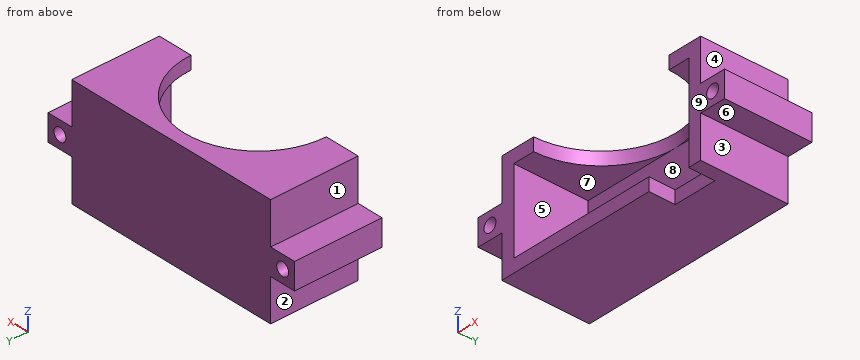
from build123d import *

# Parameters (mm, degrees)
SKETCH1_W           = 50
SKETCH1_H           = 25.18
BOSS_EXTRUDE1_DEPTH = 20
SKETCH6_W           = 44
SKETCH6_H           = 19.18
CUT_EXTRUDE4_DEPTH  = 17
CUT_EXTRUDE5_DEPTH  = 3
SKETCH8_W           = 10
SKETCH8_H           = 6
CUT_EXTRUDE6_DEPTH  = 17
SKETCH9_W           = 6
SKETCH9_H           = 6
SKETCH9_R           = 1.5
BOSS_EXTRUDE2_DEPTH = 20


with BuildPart() as part:
    # Sketch1 → Boss-Extrude1 (new body)
    with BuildSketch(Plane(origin=(0, 0, 0), x_dir=(1, 0, 0), z_dir=(0, 1, 0))):
        Rectangle(SKETCH1_W, SKETCH1_H)
    extrude(amount=BOSS_EXTRUDE1_DEPTH)

    # Sketch6 → Cut-Extrude4 (cut)
    with BuildSketch(Plane.XZ):
        Rectangle(SKETCH6_W, SKETCH6_H)
    extrude(amount=-CUT_EXTRUDE4_DEPTH, mode=Mode.SUBTRACT)

    # Sketch7 → Cut-Extrude5 (cut)
    with BuildSketch(Plane.XY.offset(12.59)):
        with BuildLine():
            Line((-17, 0), (17, 0))
            ThreePointArc((17, 0), (0, 17), (-17, 0))
        make_face()
    extrude(amount=-CUT_EXTRUDE5_DEPTH, mode=Mode.SUBTRACT)

    # Sketch8 → Cut-Extrude6 (cut)
    with BuildSketch(Plane(origin=(0, 0, -12.59), x_dir=(-1, 0, 0), z_dir=(0, 0, -1))):
        with Locations((-17, 3)):
            Rectangle(SKETCH8_W, SKETCH8_H)
    extrude(amount=-CUT_EXTRUDE6_DEPTH, mode=Mode.SUBTRACT)

    # Sketch9 → Boss-Extrude2 (add)
    with BuildSketch(Plane(origin=(0, 20, 0), x_dir=(1, 0, 0), z_dir=(0, 1, 0))):
        with Locations((28, 0)):
            Rectangle(SKETCH9_W, SKETCH9_H)
        with Locations((28, 0)):
            Circle(SKETCH9_R, mode=Mode.SUBTRACT)
        with Locations((-28, 0)):
            Rectangle(SKETCH9_W, SKETCH9_H)
        with Locations((-28, 0)):
            Circle(SKETCH9_R, mode=Mode.SUBTRACT)
    extrude(amount=-BOSS_EXTRUDE2_DEPTH)


solid = part.part
Here's how the part is built. I have some questions about the finished solid (model axes, mm). Face numbers are marked on the shaded views. A direction names the side the tool comes from. Round coordinates to 2 decimals unless told otherwise and drop trailing zeros. Loops run counter-clockwise (first coordinate to the right, second up) from the corner with the lowest first, then second, coordinate; pieces in that order, holes last. Notation, with made-up numbers: (57.5, 68) - (66.5, 68) arc R21 cw to (66.5, 72) - close; hole circle Ø2 at (61, 0). An arc over 180 degrees is marked (long way). One line per question, with ' | ' between items. Start each with the question number.
Q1. I want a section at A-A (x = -28). Write out the boundary of the cut face in (y, z).
Q2. I want a section at C-C (y = 2). Write out the boundary of the cut face in (x, z), then the cut area to 3 significant figures.
Q3. I want a section at B-B (z = 0). Write out the boundary of the cut face in (x, y), then the cut area to 3 significant figures.
Q4. Please list where these lines run through material, in increasing order: line 1 (X direction, y = 14.25, z = 0); line 2 (Z direction, x = 20, y = 8); line 3 (Z direction, x = 28, y = 11.75). Write a range as [from, to].
Q5. We'd pull the mould along Z, two halves only. Please class the marked faces 6, 7, 8 and 9: +Z half, -Z half, draft (parallel to the pull), parting line (faces both ways), or undercut.
Q6. Will these pins go through, and if not, where does the flat tip stop? pin 1 (6.5 mm diameter, centred on x = 29, y = 14, fed in from +Z); pin 2 (0.9 mm diameter, centred on x = 15, z = -11, fed in from -Y); pin 3 (8 mm diameter, centred on x = 6, y = 6.5, fed in from +Z); pin 4 (2.5 mm diameter, centred on x = -28, z = 0, fed in from +Y).
Q7. I want a section at D-D (z = 8.5). Write out the boundary of the cut face in (x, y), then the cut area to 3 significant figures.
Q8. For the marked faces 1, 2, 3, 4 and 5, which set-ups out of +Z, -Z, +X, -X, +Y, -Y let a thin tool reach every point of the face, with its end or its side?
Response values:
1) outline: (0, -3) - (20, -3) - (20, -1.5) - (0, -1.5) - close; (0, 1.5) - (20, 1.5) - (20, 3) - (0, 3) - close
2) outline: (-31, -3) - (-25, -3) - (-25, -12.59) - (12, -12.59) - (12, -9.59) - (-22, -9.59) - (-22, 9.59) - (-16.88, 9.59) - (-16.88, 12.59) - (-25, 12.59) - (-25, 3) - (-31, 3) - close; (16.88, 9.59) - (22, 9.59) - (22, -12.59) - (25, -12.59) - (25, -3) - (31, -3) - (31, 3) - (25, 3) - (25, 12.59) - (16.88, 12.59) - close; hole circle Ø3 at (-28, 0); hole circle Ø3 at (28, 0) | area: 342 mm²
3) outline: (-31, 0) - (-29.5, 0) - (-29.5, 20) - (-31, 20) - close; (-26.5, 0) - (-22, 0) - (-22, 17) - (22, 17) - (22, 0) - (26.5, 0) - (26.5, 20) - (-26.5, 20) - close; (29.5, 0) - (31, 0) - (31, 20) - (29.5, 20) - close | area: 372 mm²
4) line 1: x = [-31, -29.5], [-26.5, -22], [22, 26.5], [29.5, 31] | line 2: z = [-12.59, -9.59], [9.59, 12.59] | line 3: z = [-3, -1.5], [1.5, 3]
5) face 6: -Z half | face 7: undercut | face 8: undercut | face 9: draft
6) pin 1: stops at z = 3 | pin 2: stops at y = 6 | pin 3: stops at z = -9.59 | pin 4: passes through
7) outline: (-25, 0) - (-22, 0) - (-22, 17) - (22, 17) - (22, 0) - (25, 0) - (25, 20) - (-25, 20) - close | area: 252 mm²
8) face 1: +Z, -X, +Y, -Y | face 2: -Z, -X, +Y, -Y | face 3: -Z, +X, +Y, -Y | face 4: +Z, +X, +Y, -Y | face 5: -Y
